For this review, take the finished solid that the model builds, in its own axes (mm). Face numbers are marked on the shaded views. A direction names the side the tool comes from. Give positions to 0.01 mm unless a question says otherwise; leave off trailing zeros. Order: outer loops, then holes, each group sorted by start corner. A loop starts at its lowest first (then second) coordinate and runs counter-clockwise, first axis right, second up. Notation, with made-up numbers: M 62.5,33.25 L 104.5,33.25 A18 cw 104.5,51.25 Z; hole C 39.25,-18.75 d8. An arc over 180 degrees is marked long. Answer as CSV lines item,"result". Start each with the question number.
1. We need section A-A, the plane y = 0. Give the boundary of the cut face in (x, z), and give its area (3 significant figures).
2. We need section B-B, the plane x = 13. Give the boundary of the cut face in (y, z).
3. For line 1 along X through (y, z) = (0.5, 15); line 2 along X through (y, z) = (0, 1.05), list the stretches that pass through material, from the lowest coordinate up.
4. We need section D-D, the plane x = 29. Give the boundary of the cut face in (y, z).
5. Clearance check with flat-ended pins moving along their axes: P1, Ø2, axis at y = -3.5, z = 5.5, coming from the +X side; P2, Ø5, axis at x = 32.5, y = 9.5, coming from the +Z side. State where each tip first meets the part, or that it passes through.
6. We need section C-C, the plane y = 4. Give the boundary of the cut face in (x, z), and give its area (3 significant figures).
7. Machinability: for the marked faces 1 and 2, which of the approach directions +Z, -Z, +X, -X, +Y, -Y give a long, thin tool a straight path to every point of the face, cutting with its end or side? Answer none if there is none.
from build123d import *

# Parameters (mm, degrees)
EXTRUDE_THIN1_START = -19.05
EXTRUDE_THIN1_DEPTH = 38.1
SKETCH4_R           = 2.0828
EXTRUDE3_DEPTH      = 57.145492036


# Read off the part's stored shape, not the designer's step: Extrude-Thin1
with BuildPart() as part:
    # Extrude-Thin1 outline → Extrude-Thin1 (new body)
    with BuildSketch(Plane(origin=(0, 0, 0), x_dir=(1, 0, 0), z_dir=(0, 1, 0)).offset(EXTRUDE_THIN1_START)):
        with BuildLine():
            Line((2.286, -1.524), (38.1, -1.524))
            Line((38.1, -1.524), (38.1, 0))
            Line((38.1, 0), (2.286, 0))
            ThreePointArc((2.286, 0), (0.669553898, -0.669553898), (0, -2.286))
            Line((0, -2.286), (0, -38.1))
            Line((0, -38.1), (1.524, -38.1))
            Line((1.524, -38.1), (1.524, -2.286))
            ThreePointArc((1.524, -2.286), (1.747184633, -1.747184633), (2.286, -1.524))
        make_face()
    extrude(amount=EXTRUDE_THIN1_DEPTH)

    # Sketch4 → Extrude3 (cut, through all)
    with BuildSketch(Plane(origin=(1.524, 0, 0), x_dir=(0, 0, -1), z_dir=(1, 0, 0))):
        with Locations((-28.575, 0)):
            Circle(SKETCH4_R)
        with Locations((-14.2748, 12.7)):
            Circle(SKETCH4_R)
        with Locations((-14.2748, -12.7)):
            Circle(SKETCH4_R)
    extrude3 = extrude(amount=-EXTRUDE3_DEPTH, mode=Mode.SUBTRACT)

    # Mirror1: Extrude3 across plane
    add(extrude3.mirror(Plane(origin=(0, 0, 0), x_dir=(0.7071067811865465, 0, 0.7071067811865486), z_dir=(-0.7071067811865488, 0, 0.7071067811865464))), mode=Mode.SUBTRACT)


solid = part.part
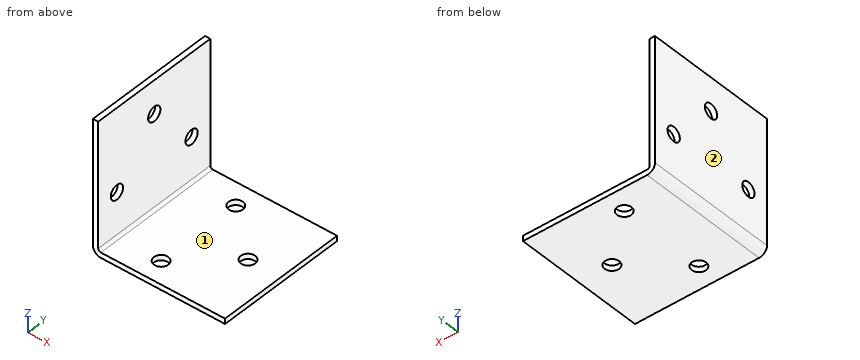
Result set:
1,outline,"M 0,2.29 A2.29 ccw 2.29,0 L 26.49,0 L 26.49,1.52 L 2.29,1.52 A0.76 cw 1.52,2.29 L 1.52,26.49 L 0,26.49 Z; M 0,30.66 L 1.52,30.66 L 1.52,38.1 L 0,38.1 Z; M 30.66,0 L 38.1,0 L 38.1,1.52 L 30.66,1.52 Z"
1,area,"100 mm2"
2,outline,"M -19.05,0 L -14.35,0 L -14.35,1.52 L -19.05,1.52 Z; M -11.05,0 L 11.05,0 L 11.05,1.52 L -11.05,1.52 Z; M 14.35,0 L 19.05,0 L 19.05,1.52 L 14.35,1.52 Z"
3,line 1,"0 to 1.52"
3,line 2,"0.36 to 26.49, 30.66 to 38.1"
4,outline,"M -19.05,0 L -2.04,0 L -2.04,1.52 L -19.05,1.52 Z; M 2.04,0 L 19.05,0 L 19.05,1.52 L 2.04,1.52 Z"
5,P1,"x = 1.52"
5,P2,"z = 1.52"
6,outline,"M 0,2.29 A2.29 ccw 2.29,0 L 38.1,0 L 38.1,1.52 L 2.29,1.52 A0.76 cw 1.52,2.29 L 1.52,38.1 L 0,38.1 Z"
6,area,"113 mm2"
7,face 1,"+Z, +X, +Y, -Y"
7,face 2,"+Z, -Z, -X, +Y, -Y"
